```python
from build123d import *

# Parameters (mm, degrees)
PAD002_DEPTH = 10
PAD001_DEPTH = 1
PAD007_DEPTH = 4


with BuildPart() as body002_bot:
    # Sketch002 → Pad002 (new body)
    with BuildSketch(Plane.XZ):
        with BuildLine():
            ThreePointArc((14.183335, 20), (24.999984, 7), (35.816645, 19.999991))
            Line((40.816645, 19.999991), (35.816645, 19.999991))
            Line((50, 0), (40.816645, 19.999991))
            Line((0, 0), (50, 0))
            Line((9.183335, 20), (0, 0))
            Line((14.183335, 20), (9.183335, 20))
        make_face()
    extrude(amount=-PAD002_DEPTH)


with BuildPart() as body001_bot:
    # Sketch001 → Pad001 (new body)
    with BuildSketch(Plane.XZ):
        with BuildLine():
            ThreePointArc((16.841546, 20), (24.999965, 9.6), (33.158414, 19.999976))
            Line((38.158414, 19.999976), (33.158414, 19.999976))
            Line((50, 0), (38.158414, 19.999976))
            Line((0, 0), (50, 0))
            Line((11.841546, 20), (0, 0))
            Line((16.841546, 20), (11.841546, 20))
        make_face()
    extrude(amount=-PAD001_DEPTH)

    # Boolean001: union Body002_bot
    add(body002_bot.part)

    # Sketch007 → Pad007 (join)
    with BuildSketch(Plane.XZ):
        Polygon((11, -4), (11, 4.332914), (39, 4.332914), (39, -4), (35, -4), (35, 0), (15, 0), (15, -4), align=None)
    extrude(amount=-PAD007_DEPTH)


solid = body001_bot.part
```
Design review of the part built by this model. Coordinates are the model's own, in mm. A direction names the side the tool comes from. Give positions to 0.01 mm unless a question says otherwise; leave off trailing zeros. Order: outer loops, then holes, each group sorted by start corner. A loop starts at its lowest first (then second) coordinate and runs counter-clockwise, first axis right, second up. Notation, with made-up numbers: (12, 47) -> (27, 47) arc R26 ccw to (27, 61) -> close; hole circle Ø1 at (-19, 70). An arc over 180 degrees is marked (long way). Write item = value, one per line. Start each with the question number.
(1) To check wall thickness, follow line 1 along Z through (x, y) = (10, 7); line 2 along X through (y, z) = (4.5, 15); line 3 along Y through (x, z) = (16, 16.5). State the ranges of each line that lie inside material, in increasing order.
(2) We need section C-C on y = 1.5. Write out the cut boundary in (x, z).
(3) For pin 1 (1.2 mm diameter, centred on x = 36, z = -3, fed in from +Y); pin 2 (2 mm diameter, centred on y = 1.5, z = -2, fed in from +X); pin 3 (1.2 mm diameter, centred on y = 2, z = -1, fed in from -X), all flat-tipped, find the tip position at first contact; note any pin that passes through.
(4) Mouldability with a two-part tool opening along X and no side actions: class faces 5 (the face through (11, 2, -2)), 6 (the face through (34.5, 0.5, 20)), 7 (the face through (45.473, 4.93, 9.86)), 8 (the face through (15, 2, -2)) as +X half, -X half, draft (parallel to the pull), parting line (faces both ways), or undercut.
(5) We need section D-D on z = 17.75. Write out the cut boundary in (x, y).
(6) We need section B-B on x = 12.5. Write out the cut boundary in (y, z).
(7) For faces 1 (the face through (25, 10, 6)), 2 (the face through (35, 2, -2)), 3 (the face through (39, 2, -2)), 4 (the face through (37, 4, -2)), list the 3-axis set-ups (+Z, -Z, +X, -X, +Y, -Y) from which the entire face can be reached by the end or side of a thin tool; tool diameter is ignored.
(8) We need section A-A on z = -1.75. Write out the cut boundary in (x, y).
Numbers:
q1.line_1 = 0 to 20
q1.line_2 = 6.89 to 14.42, 35.58 to 43.11
q1.line_3 = 0 to 1
q2.outline = (0, 0) -> (11, 0) -> (11, -4) -> (15, -4) -> (15, 0) -> (35, 0) -> (35, -4) -> (39, -4) -> (39, 0) -> (50, 0) -> (40.82, 20) -> (35.82, 20) arc R11 cw (long way) to (14.18, 20) -> (9.18, 20) -> close
q3.pin_1 = 4
q3.pin_2 = 39
q3.pin_3 = 11
q4.face_5 = -X half
q4.face_6 = draft
q4.face_7 = +X half
q4.face_8 = undercut
q5.outline = (8.15, 0) -> (16.6, 0) -> (16.6, 1) -> (14, 1) -> (14, 10) -> (8.15, 10) -> close; (33.4, 0) -> (41.85, 0) -> (41.85, 10) -> (36, 10) -> (36, 1) -> (33.4, 1) -> close
q6.outline = (0, -4) -> (4, -4) -> (4, 0) -> (10, 0) -> (10, 20) -> (0, 20) -> close
q7.face_1 = +Z, -Z, +X, -X, +Y
q7.face_2 = -Z, +Y, -Y
q7.face_3 = -Z, +X, +Y, -Y
q7.face_4 = -Z, +X, -X, +Y
q8.outline = (11, 0) -> (15, 0) -> (15, 4) -> (11, 4) -> close; (35, 0) -> (39, 0) -> (39, 4) -> (35, 4) -> close
